```python
from build123d import *

# Parameters (mm, degrees)
SKETCH1_R                = 20
BOSS_EXTRUDE1_DEPTH      = 3.5
SKETCH2_R                = 35
SKETCH2_R_2              = 20
SKETCH2_R_3              = 2.8
BOSS_EXTRUDE2_DEPTH      = 6
BOSS_EXTRUDE3_DEPTH      = 2
BOSS_EXTRUDE3_DEPTH_BACK = 6
SKETCH4_R                = 2.9
SKETCH5_R                = 5
BOSS_EXTRUDE4_DEPTH      = 3
CUT_EXTRUDE1_START       = -10
SKETCH3_R                = 20
CUT_EXTRUDE1_DEPTH       = 10
SKETCH12_R               = 72.135852014
CUT_EXTRUDE2_DEPTH       = 22
FILLET1_R                = 10
CUT_EXTRUDE4_START       = -2
SKETCH15_R               = 5
SKETCH15_R_2             = 20
CUT_EXTRUDE4_DEPTH       = 2


with BuildPart() as part:
    # Sketch1 → Boss-Extrude1 (new body)
    with BuildSketch(Plane(origin=(0, 0, 0), x_dir=(1, 0, 0), z_dir=(0, 1, 0))):
        with Locations(Location((0, 0, 0), (0, 0, 270))):
            Circle(SKETCH1_R)
    extrude(amount=BOSS_EXTRUDE1_DEPTH)

    # Sketch2 → Boss-Extrude2 (add)
    with BuildSketch(Plane(origin=(0, 0, 0), x_dir=(1, 0, 0), z_dir=(0, 1, 0))):
        with Locations(Location((0, 0, 0), (0, 0, 270))):
            Circle(SKETCH2_R)
        with Locations(Location((0, 0, 0), (0, 0, 270))):
            Circle(SKETCH2_R_2, mode=Mode.SUBTRACT)
        with Locations(Location((0, 28.3, 0), (0, 0, 270))):
            Circle(SKETCH2_R_3, mode=Mode.SUBTRACT)
        with Locations(Location((24.508518927, -14.15, 0), (0, 0, 270))):
            Circle(SKETCH2_R_3, mode=Mode.SUBTRACT)
        with Locations(Location((-24.508518927, -14.15, 0), (0, 0, 270))):
            Circle(SKETCH2_R_3, mode=Mode.SUBTRACT)
    extrude(amount=BOSS_EXTRUDE2_DEPTH)

    # Sketch4 → Boss-Extrude3 (add, two sides: drawn at the far end of the back side and taken through both)
    with BuildSketch(Plane.XZ.offset(-BOSS_EXTRUDE3_DEPTH_BACK)):
        with Locations(Location((-24.508518927, 14.15, 0), (0, 0, 270))):
            Circle(SKETCH4_R)
        with Locations(Location((24.508518927, 14.15, 0), (0, 0, 270))):
            Circle(SKETCH4_R)
        with Locations(Location((0, -28.3, 0), (0, 0, 270))):
            Circle(SKETCH4_R)
    extrude(amount=BOSS_EXTRUDE3_DEPTH + BOSS_EXTRUDE3_DEPTH_BACK)

    # Sketch5 → Boss-Extrude4 (add)
    with BuildSketch(Plane(origin=(0, 6, 0), x_dir=(1, 0, 0), z_dir=(0, 1, 0))):
        with Locations((-30.453629482, -17.250404383)):
            Circle(SKETCH5_R)
        with Locations((0.28752632, 34.99881896)):
            Circle(SKETCH5_R)
        with Locations((30.166103162, -17.748414577)):
            Circle(SKETCH5_R)
    extrude(amount=-BOSS_EXTRUDE4_DEPTH)

    # Sketch3 → Cut-Extrude1 (cut)
    with BuildSketch(Plane(origin=(0, 3.5, 0), x_dir=(1, 0, 0), z_dir=(0, 1, 0)).offset(CUT_EXTRUDE1_START)):
        with Locations(Location((0, 0, 0), (0, 0, 270))):
            Circle(SKETCH3_R)
    extrude(amount=CUT_EXTRUDE1_DEPTH, mode=Mode.SUBTRACT)

    # Sketch12 → Cut-Extrude2 (cut)
    with BuildSketch(Plane(origin=(0, 6, 0), x_dir=(1, 0, 0), z_dir=(0, 1, 0))):
        Circle(SKETCH12_R)
        Polygon((0, 50), (-43.301270189, -25), (43.301270189, -25), align=None, mode=Mode.SUBTRACT)
    extrude(amount=-CUT_EXTRUDE2_DEPTH, mode=Mode.SUBTRACT)

    # Fillet1
    # the kernel refuses this fillet: 10 mm, written as the material it takes off along each edge
    with BuildSketch(Plane(origin=(-24.494897428, 19.2960859, 25), x_dir=(1, 0, 0), z_dir=(0, -1, 0))) as fillet1_piece_1_section:
        with BuildLine():
            CenterArc((4.494897428, -10), FILLET1_R, 90, 53.130102354)
            ThreePointArc((-3.505102572, -4), (-1.828638885, -1.933326291), (0, 0))
            Line((0, 0), (4.494897428, 0))
        make_face()
    fillet1_piece_1 = extrude(amount=32.5921718, mode=Mode.PRIVATE)
    fillet1_piece_1 = fillet1_piece_1 - Plane(origin=(-30.453629482, 4.5, 17.250404383), x_dir=(1, 0, 0), z_dir=(0, 1, 0)) * Cylinder(5, 84, mode=Mode.PRIVATE)
    add(fillet1_piece_1, mode=Mode.SUBTRACT)
    with BuildSketch(Plane(origin=(-24.494897428, 19.2960859, 25), x_dir=(1, 0, 0), z_dir=(0, -1, 0))) as fillet1_piece_2_section:
        with BuildLine():
            CenterArc((4.494897428, -10), FILLET1_R, 90, 53.130102354)
            ThreePointArc((-3.505102572, -4), (-1.828638885, -1.933326291), (0, 0))
            Line((0, 0), (4.494897428, 0))
        make_face()
    fillet1_piece_2 = extrude(amount=32.5921718, mode=Mode.PRIVATE)
    fillet1_piece_2 = split(fillet1_piece_2, bisect_by=Plane(origin=(-27.761621835, 3, 21.309124186), z_dir=(0, -1, 0)), keep=Keep.TOP, mode=Mode.PRIVATE)
    add(fillet1_piece_2, mode=Mode.SUBTRACT)
    with BuildSketch(Plane(origin=(24.494897428, 19.2960859, 25), x_dir=(-1, 0, 0), z_dir=(0, -1, 0))) as fillet1_piece_3_section:
        with BuildLine():
            CenterArc((4.494897428, 10), FILLET1_R, 216.869897646, 53.130102354)
            ThreePointArc((-3.505102572, 4), (-1.828638885, 1.933326291), (0, 0))
            Line((0, 0), (4.494897428, 0))
        make_face()
    fillet1_piece_3 = extrude(amount=32.5921718, mode=Mode.PRIVATE)
    fillet1_piece_3 = fillet1_piece_3 - Plane(origin=(30.166103162, 4.5, 17.748414577), x_dir=(1, 0, 0), z_dir=(0, 1, 0)) * Cylinder(5, 84, mode=Mode.PRIVATE)
    add(fillet1_piece_3, mode=Mode.SUBTRACT)
    with BuildSketch(Plane(origin=(24.494897428, 19.2960859, 25), x_dir=(-1, 0, 0), z_dir=(0, -1, 0))) as fillet1_piece_4_section:
        with BuildLine():
            CenterArc((4.494897428, 10), FILLET1_R, 216.869897646, 53.130102354)
            ThreePointArc((-3.505102572, 4), (-1.828638885, 1.933326291), (0, 0))
            Line((0, 0), (4.494897428, 0))
        make_face()
    fillet1_piece_4 = extrude(amount=32.5921718, mode=Mode.PRIVATE)
    fillet1_piece_4 = split(fillet1_piece_4, bisect_by=Plane(origin=(27.488157838, 3, 21.643747381), z_dir=(0, -1, 0)), keep=Keep.TOP, mode=Mode.PRIVATE)
    add(fillet1_piece_4, mode=Mode.SUBTRACT)
    with BuildSketch(Plane(origin=(-9.403186381, 19.2960859, -33.713203436), x_dir=(-0.5000000000000003, 0, 0.8660254037844386), z_dir=(0, -1, 0))) as fillet1_piece_5_section:
        with BuildLine():
            CenterArc((4.494897428, -10), FILLET1_R, 90, 53.130102354)
            ThreePointArc((-3.505102572, -4), (-1.828638885, -1.933326291), (0, 0))
            Line((0, 0), (4.494897428, 0))
        make_face()
    fillet1_piece_5 = extrude(amount=32.5921718, mode=Mode.PRIVATE)
    fillet1_piece_5 = fillet1_piece_5 - Plane(origin=(0.28752632, 4.5, -34.99881896), x_dir=(1, 0, 0), z_dir=(0, 1, 0)) * Cylinder(5, 84, mode=Mode.PRIVATE)
    add(fillet1_piece_5, mode=Mode.SUBTRACT)
    with BuildSketch(Plane(origin=(-9.403186381, 19.2960859, -33.713203436), x_dir=(-0.5000000000000003, 0, 0.8660254037844386), z_dir=(0, -1, 0))) as fillet1_piece_6_section:
        with BuildLine():
            CenterArc((4.494897428, -10), FILLET1_R, 90, 53.130102354)
            ThreePointArc((-3.505102572, -4), (-1.828638885, -1.933326291), (0, 0))
            Line((0, 0), (4.494897428, 0))
        make_face()
    fillet1_piece_6 = extrude(amount=32.5921718, mode=Mode.PRIVATE)
    fillet1_piece_6 = split(fillet1_piece_6, bisect_by=Plane(origin=(-4.57343196, 3, -34.696831852), z_dir=(0, -1, 0)), keep=Keep.TOP, mode=Mode.PRIVATE)
    add(fillet1_piece_6, mode=Mode.SUBTRACT)
    with BuildSketch(Plane(origin=(-33.898083809, 19.2960859, 8.713203436), x_dir=(0.32181469455231854, 0, 0.9468026734067654), z_dir=(0, -1, 0))) as fillet1_piece_7_section:
        with BuildLine():
            CenterArc((4.558658023, -9.971095222), FILLET1_R, 85.642603122, 53.130102354)
            Line((-2.962352352, -3.380617019), (0, 0))
            ThreePointArc((0, 0), (2.65921718, 0.101166725), (5.31843436, 0))
        make_face()
    fillet1_piece_7 = extrude(amount=32.5921718, mode=Mode.PRIVATE)
    fillet1_piece_7 = fillet1_piece_7 - Plane(origin=(-30.453629482, 4.5, 17.250404383), x_dir=(1, 0, 0), z_dir=(0, 1, 0)) * Cylinder(5, 87, mode=Mode.PRIVATE)
    add(fillet1_piece_7, mode=Mode.SUBTRACT)
    with BuildSketch(Plane(origin=(-33.898083809, 19.2960859, 8.713203436), x_dir=(0.32181469455231854, 0, 0.9468026734067654), z_dir=(0, -1, 0))) as fillet1_piece_8_section:
        with BuildLine():
            CenterArc((4.558658023, -9.971095222), FILLET1_R, 85.642603122, 53.130102354)
            Line((-2.962352352, -3.380617019), (0, 0))
            ThreePointArc((0, 0), (2.65921718, 0.101166725), (5.31843436, 0))
        make_face()
    fillet1_piece_8 = extrude(amount=32.5921718, mode=Mode.PRIVATE)
    fillet1_piece_8 = split(fillet1_piece_8, bisect_by=Plane(origin=(-32.488113984, 3, 12.9835693), z_dir=(0, -1, 0)), keep=Keep.TOP, mode=Mode.PRIVATE)
    add(fillet1_piece_8, mode=Mode.SUBTRACT)
    with BuildSketch(Plane(origin=(33.898083809, 19.2960859, 8.713203436), x_dir=(-0.5000000000000012, 0, -0.8660254037844382), z_dir=(0, -1, 0))) as fillet1_piece_9_section:
        with BuildLine():
            CenterArc((4.494897428, -10), FILLET1_R, 90, 53.130102354)
            ThreePointArc((-3.505102572, -4), (-1.828638885, -1.933326291), (0, 0))
            Line((0, 0), (4.494897428, 0))
        make_face()
    fillet1_piece_9 = extrude(amount=32.5921718, mode=Mode.PRIVATE)
    fillet1_piece_9 = fillet1_piece_9 - Plane(origin=(30.166103162, 4.5, 17.748414577), x_dir=(1, 0, 0), z_dir=(0, 1, 0)) * Cylinder(5, 84, mode=Mode.PRIVATE)
    add(fillet1_piece_9, mode=Mode.SUBTRACT)
    with BuildSketch(Plane(origin=(33.898083809, 19.2960859, 8.713203436), x_dir=(-0.5000000000000012, 0, -0.8660254037844382), z_dir=(0, -1, 0))) as fillet1_piece_10_section:
        with BuildLine():
            CenterArc((4.494897428, -10), FILLET1_R, 90, 53.130102354)
            ThreePointArc((-3.505102572, -4), (-1.828638885, -1.933326291), (0, 0))
            Line((0, 0), (4.494897428, 0))
        make_face()
    fillet1_piece_10 = extrude(amount=32.5921718, mode=Mode.PRIVATE)
    fillet1_piece_10 = split(fillet1_piece_10, bisect_by=Plane(origin=(32.335053795, 3, 13.387707666), z_dir=(0, -1, 0)), keep=Keep.TOP, mode=Mode.PRIVATE)
    add(fillet1_piece_10, mode=Mode.SUBTRACT)
    with BuildSketch(Plane(origin=(9.403186381, 19.2960859, -33.713203436), x_dir=(-0.9808625148174394, 0, -0.19470163590994477), z_dir=(0, -1, 0))) as fillet1_piece_11_section:
        with BuildLine():
            CenterArc((4.558658023, -9.971095222), FILLET1_R, 85.642603122, 53.130102354)
            Line((-2.962352352, -3.380617019), (0, 0))
            ThreePointArc((0, 0), (2.65921718, 0.101166725), (5.31843436, 0))
        make_face()
    fillet1_piece_11 = extrude(amount=32.5921718, mode=Mode.PRIVATE)
    fillet1_piece_11 = fillet1_piece_11 - Plane(origin=(0.28752632, 4.5, -34.99881896), x_dir=(1, 0, 0), z_dir=(0, 1, 0)) * Cylinder(5, 87, mode=Mode.PRIVATE)
    add(fillet1_piece_11, mode=Mode.SUBTRACT)
    with BuildSketch(Plane(origin=(9.403186381, 19.2960859, -33.713203436), x_dir=(-0.9808625148174394, 0, -0.19470163590994477), z_dir=(0, -1, 0))) as fillet1_piece_12_section:
        with BuildLine():
            CenterArc((4.558658023, -9.971095222), FILLET1_R, 85.642603122, 53.130102354)
            Line((-2.962352352, -3.380617019), (0, 0))
            ThreePointArc((0, 0), (2.65921718, 0.101166725), (5.31843436, 0))
        make_face()
    fillet1_piece_12 = extrude(amount=32.5921718, mode=Mode.PRIVATE)
    fillet1_piece_12 = split(fillet1_piece_12, bisect_by=Plane(origin=(4.999956146, 3, -34.627316681), z_dir=(0, -1, 0)), keep=Keep.TOP, mode=Mode.PRIVATE)
    add(fillet1_piece_12, mode=Mode.SUBTRACT)

    # Sketch15 → Cut-Extrude4 (cut)
    with BuildSketch(Plane(origin=(0, 6, 0), x_dir=(1, 0, 0), z_dir=(0, 1, 0)).offset(CUT_EXTRUDE4_START)):
        with Locations((0, 20)):
            Circle(SKETCH15_R)
        with Locations(Location((0, 0, 0), (0, 0, 104.361511563))):
            Circle(SKETCH15_R_2)
        with Locations((-17.320508076, -10)):
            Circle(SKETCH15_R)
        with Locations((17.320508076, -10)):
            Circle(SKETCH15_R)
    extrude(amount=CUT_EXTRUDE4_DEPTH, mode=Mode.SUBTRACT)


solid = part.part
```
Source: CAD feature listing. Evaluate the final solid. Frame: model axes, mm. A direction names the side the tool comes from. Give positions to 0.01 mm unless a question says otherwise; leave off trailing zeros. Write each loop counter-clockwise with the first axis right and the second up, starting at its lowest first coordinate (ties: lowest second). Pieces come first, ordered by that corner, then holes. Notation, with made-up numbers: (45.25, 1.25) - (50.25, 1.25) arc R22 ccw to (50.25, 24.25) - close; hole circle Ø7 at (72.5, 10.5). An arc over 180 degrees is marked (long way). One line per item, written item: value. Start each with the question number.
Q1. Draft query along Z for faces 4 (the face through (0, 1, -35)), 5 (the face through (0, 5, -25)), 6 (the face through (24.53, 3.042, 23.915)). Return one class per face: +Z half, -Z half, draft (parallel to the pull), parting line (faces both ways), or undercut.
Q2. First-contact query: pin 1 Ø1.7 at (x, z) = (-0.5, -22) entering from +Y; pin 2 Ø6 at (x, z) = (0, -20) entering from -Y; pin 3 Ø4.5 at (x, z) = (1.5, -38) entering from -Y. Flat tips, straight axial feed; report the tip coordinate or a pass-through.
Q3. Section query C-C, the plane z = -27. Return the cut outline in (x, y).
Q4. Material intervals for probe 1 along Z at (x, y) = (0, 3.9); probe 2 along Z at (x, y) = (-0.5, 1.5); probe 3 along Y at (x, z) = (-19, 9), sorted ascending. Write a range as from..to.
Q5. Section query B-B, the plane x = 0. Return the cut outline in (y, z), then the cut area to 3 significant figures.
Q6. Section query A-A, the plane z = -15. Return the cut outline in (x, y).
Q7. Set-up query: faces 1 (the face through (32, 3, 19)), 2 (the face through (19, 4, 11)), 3 (the face through (26.468, -0.986, 16.287)). Return all of +Z, -Z, +X, -X, +Y, -Y with unobstructed straight access to the full face (end or side cutting, diameter ignored); none if empty.
Q8. Section query D-D, the plane x = -17. Return the cut outline in (y, z).
Answer:
1. face 4: -Z half
1. face 5: undercut
1. face 6: +Z half
2. pin 1: stops at y = 4
2. pin 2: stops at y = 0
2. pin 3: stops at y = 3
3. outline: (-13.28, 0) - (-2.59, 0) - (-2.59, -2) - (2.59, -2) - (2.59, 0) - (13.28, 0) - (13.28, 6) - (-13.28, 6) - close
4. probe 1: z = -39.99..-20, 20..25
4. probe 2: z = -35..-19.99, 19.99..25
4. probe 3: y = 0..4
5. outline: (-2, -31.2) - (0, -31.2) - (0, -35) - (3, -35) - (3, -39.99) - (6, -39.99) - (6, -25) - (4, -25) - (4, -20) - (0, -20) - (0, -25.4) - (-2, -25.4) - close; (0, 20) - (6, 20) - (6, 25) - (0, 25) - close
5. area: 137 mm2
6. outline: (-20.21, 0) - (-13.23, 0) - (-13.23, 6) - (-20.21, 6) - close; (13.23, 0) - (20.21, 0) - (20.21, 6) - (13.23, 6) - close
7. face 1: +Z, +X, -Y
7. face 2: +Y
7. face 3: -Y
8. outline: (0, -20.56) - (6, -20.56) - (6, -10.54) - (0, -10.54) - close; (0, 10.54) - (4, 10.54) - (4, 14.99) - (6, 14.99) - (6, 25) - (0, 25) - close
